For this review, take the finished solid that the model builds, in its own axes (mm). A direction names the side the tool comes from. Round coordinates to 2 decimals unless told otherwise and drop trailing zeros. Loops run counter-clockwise (first coordinate to the right, second up) from the corner with the lowest first, then second, coordinate; pieces in that order, holes last.
1. Tool access review of faces 1 (the cylindrical face through (-1.856, 10.14, -2.42)), 2 (the cylindrical face through (1.01, 25.07, 0.65)): name each direction out of +Z, -Z, +X, -X, +Y, -Y from which nothing blocks a thin tool from reaching the whole face with its end or side.
2. Draft analysis for pull direction X (two halves, no side actions). For faces 3 (the flat face through (-1, 20, 1)), 4 (the cylindrical face through (1.352, 14.79, 4.292)), 5 (the flat face through (-1, 30, 1)), state which applies: released by +X, released by -X, zero draft, split by the parting line, or undercut.
3. Clearance check with flat-ended pins moving along their axes: pin 1 Ø1 at (x, z) = (-0.5, 0) entering from -Y; pin 2 Ø3 at (x, z) = (0, 1) entering from -Y. State where each tip first meets the part, or that it passes through.
4. Consider section C-C on z = 2.5. State the section outline as (x, y) points, then the cut area to 3 significant figures.
5. Consider section B-B on z = 0. State the section outline as (x, y) points.
6. Consider section A-A on x = 0. State the section outline as (y, z) points.
7. To check wall thickness, follow line 1 along X through (y, z) = (5.75, 0); line 2 along Y through (x, z) = (-1.5, -2); line 3 along X through (y, z) = (24.25, 0). State the ranges of each line that lie inside material, in increasing order.
8. Consider section D-D on y = 6. State the section outline as (x, z) points, then the cut area to 3 significant figures.
from build123d import *

# Parameters (mm, degrees)
SKETCH1_R           = 4.5
BOSS_EXTRUDE1_DEPTH = 30
SKETCH2_R           = 3.05
CUT_EXTRUDE1_DEPTH  = 31.66757245
SKETCH3_R           = 3.05
BOSS_EXTRUDE2_DEPTH = 10
SKETCH4_R           = 1.2
CUT_EXTRUDE2_DEPTH  = 10


with BuildPart() as part:
    # Sketch1 → Boss-Extrude1 (new body)
    with BuildSketch(Plane(origin=(0, 0, 0), x_dir=(1, 0, 0), z_dir=(0, 1, 0))):
        with Locations(Location((0, 0, 0), (0, 0, 270))):
            Circle(SKETCH1_R)
    extrude(amount=BOSS_EXTRUDE1_DEPTH)

    # Sketch2 → Cut-Extrude1 (cut, through all)
    with BuildSketch(Plane(origin=(0, 30, 0), x_dir=(1, 0, 0), z_dir=(0, 1, 0))):
        with Locations(Location((0, 0, 0), (0, 0, 270))):
            Circle(SKETCH2_R)
    extrude(amount=-CUT_EXTRUDE1_DEPTH, mode=Mode.SUBTRACT)

    # Sketch3 → Boss-Extrude2 (add)
    with BuildSketch(Plane(origin=(0, 30, 0), x_dir=(1, 0, 0), z_dir=(0, 1, 0))):
        with Locations(Location((0, 0, 0), (0, 0, 270))):
            Circle(SKETCH3_R)
    extrude(amount=-BOSS_EXTRUDE2_DEPTH)

    # Sketch4 → Cut-Extrude2 (cut)
    with BuildSketch(Plane(origin=(0, 30, 0), x_dir=(1, 0, 0), z_dir=(0, 1, 0))):
        with Locations(Location((0, 0, 0), (0, 0, 270))):
            Circle(SKETCH4_R)
    extrude(amount=-CUT_EXTRUDE2_DEPTH, mode=Mode.SUBTRACT)


solid = part.part
Resolved:
1. face 1: -Y
1. face 2: +Y, -Y
2. face 3: undercut
2. face 4: split by the parting line
2. face 5: zero draft
3. pin 1: passes through
3. pin 2: stops at y = 20
4. outline: (-3.74, 0) - (-1.75, 0) - (-1.75, 20) - (1.75, 20) - (1.75, 0) - (3.74, 0) - (3.74, 30) - (-3.74, 30) - close
4. area: 155 mm2
5. outline: (-4.5, 0) - (-3.05, 0) - (-3.05, 20) - (-1.2, 20) - (-1.2, 30) - (-4.5, 30) - close; (1.2, 20) - (3.05, 20) - (3.05, 0) - (4.5, 0) - (4.5, 30) - (1.2, 30) - close
6. outline: (0, -4.5) - (30, -4.5) - (30, -1.2) - (20, -1.2) - (20, -3.05) - (0, -3.05) - close; (0, 3.05) - (20, 3.05) - (20, 1.2) - (30, 1.2) - (30, 4.5) - (0, 4.5) - close
7. line 1: x = -4.5 to -3.05, 3.05 to 4.5
7. line 2: y = 20 to 30
7. line 3: x = -4.5 to -1.2, 1.2 to 4.5
8. outline: circle Ø9 at (0, 0); hole circle Ø6.1 at (0, 0)
8. area: 34.4 mm2
